from build123d import *

# Parameters (mm, degrees)
SKETCH1_R           = 2.64
BOSS_EXTRUDE1_DEPTH = 3
SKETCH2_R           = 1.405
BOSS_EXTRUDE2_DEPTH = 7.76
FILLET1_R           = 0.2
CUT_EXTRUDE1_DEPTH  = 1.5
FILLET2_R           = 0.2
FILLET3_R           = 0.5


with BuildPart() as part:
    # Sketch1 → Boss-Extrude1 (new body)
    with BuildSketch(Plane(origin=(0, 0, 0), x_dir=(1, 0, 0), z_dir=(0, 1, 0))):
        with Locations(Location((0, 0, 0), (0, 0, 270))):
            Circle(SKETCH1_R)
    extrude(amount=BOSS_EXTRUDE1_DEPTH)

    # Sketch2 → Boss-Extrude2 (add)
    with BuildSketch(Plane.XZ):
        with Locations(Location((0, 0, 0), (0, 0, 270))):
            Circle(SKETCH2_R)
    extrude(amount=BOSS_EXTRUDE2_DEPTH)

    # Fillet1
    fillet1_edges = [part.edges().sort_by_distance(p)[0] for p in [
        (0, 0, -2.64),
        (0, 3, -2.64),
    ]]
    fillet(fillet1_edges, radius=FILLET1_R)

    # Sketch3 → Cut-Extrude1 (cut)
    with BuildSketch(Plane(origin=(0, 3, 0), x_dir=(1, 0, 0), z_dir=(0, 1, 0))):
        Polygon((1.385640646, 0), (0.692820323, 1.2), (-0.692820323, 1.2), (-1.385640646, 0), (-0.692820323, -1.2), (0.692820323, -1.2), align=None)
    extrude(amount=-CUT_EXTRUDE1_DEPTH, mode=Mode.SUBTRACT)

    # Fillet2
    fillet2_edges = [part.edges().sort_by_distance(p)[0] for p in [
        (1.039230485, 3, 0.6),
        (1.039230485, 3, -0.6),
        (0, 3, -1.2),
        (-1.039230485, 3, -0.6),
        (-1.039230485, 3, 0.6),
        (0, 3, 1.2),
    ]]
    fillet(fillet2_edges, radius=FILLET2_R)

    # Fillet3
    fillet3_edges = [part.edges().sort_by_distance(p)[0] for p in [
        (0, -7.76, 1.405),
    ]]
    fillet(fillet3_edges, radius=FILLET3_R)


solid = part.part
Geometry: final body of the model. Coordinates: model frame, mm. A direction names the side the tool comes from. Round coordinates to 2 decimals unless told otherwise and drop trailing zeros. Loops run counter-clockwise (first coordinate to the right, second up) from the corner with the lowest first, then second, coordinate; pieces in that order, holes last.
Q1. Section A-A on x = 0. Return loops of the section in (y, z) (3 decimals).
Q2. Section B-B on y = -1.25. Return loops of the section in (x, z) (3 decimals).
Q3. Pull-direction query (X, two-part tool) for faces 1 (the cylindrical face through (-1.372, -3.579, 0.305)), 2 (the flat face through (-1.034, 2.159, -0.608)), 3 (the flat face through (0, 3, 2)); classes: released by +X, released by -X, zero draft, split by the parting line, or undercut.
Q4. Pin query (flat end, axial travel): P1, Ø2, axis at y = -0.5, z = 0, coming from the -X side; P2, Ø1.2, axis at x = 0, z = 0.5, coming from the +Y side. Return the tip coordinate at first contact, or that it passes through.
Q5. Access query for faces 4 (the flat face through (0, -7.76, 0)), 5 (the flat face through (-1.1, 0, 1.1)), 6 (the cylindrical face through (-1.086, 2.943, 0.64)). Directions: +Z, -Z, +X, -X, +Y, -Y. A direction counts if a zero-diameter tool reaches every point of the face in a straight line with its end or side. Return the directions, or none.
Q6. Material intervals for L1, parallel to Y at x = 0.2, z = 1.8; L2, parallel to X at y = 2.5, z = 0.95; L3, parallel to Y at x = -0.7, z = 0.65, sorted ascending.
Evaluation:
1. outline: (-7.76, -0.905) arc R0.5 ccw to (-7.26, -1.405) - (0, -1.405) - (0, -2.44) arc R0.2 ccw to (0.2, -2.64) - (2.8, -2.64) arc R0.2 ccw to (3, -2.44) - (3, -1.4) arc R0.2 ccw to (2.8, -1.2) - (1.5, -1.2) - (1.5, 1.2) - (2.8, 1.2) arc R0.2 ccw to (3, 1.4) - (3, 2.44) arc R0.2 ccw to (2.8, 2.64) - (0.2, 2.64) arc R0.2 ccw to (0, 2.44) - (0, 1.405) - (-7.26, 1.405) arc R0.5 ccw to (-7.76, 0.905) - close
2. outline: circle Ø2.81 at (0, 0)
3. face 1: split by the parting line
3. face 2: undercut
3. face 3: zero draft
4. P1: stops at x = -2.64
4. P2: stops at y = 1.5
5. face 4: +Z, -Z, +X, -X, -Y
5. face 5: -Y
5. face 6: +Y
6. L1: y = 0 to 3
6. L2: x = -2.46 to -0.84, 0.84 to 2.46
6. L3: y = -7.76 to 1.5
